from build123d import *

# Parameters (mm, degrees)
BOSS_EXTRUDE1_DEPTH            = 7.5
M3_CLEARANCE_HOLE1_D           = 3.4
M3_CLEARANCE_HOLE1_CSINK_D     = 3.45
M3_CLEARANCE_HOLE1_CSINK_ANGLE = 90
FILLET1_R                      = 30


with BuildPart() as part:
    # Sketch1 → Boss-Extrude1 (new body)
    with BuildSketch(Plane(origin=(0, 0, 0), x_dir=(0, 0, -1), z_dir=(1, 0, 0))):
        Polygon((0, 0), (0, 45), (9.5, 45), (9.5, 9.5), (40, 9.5), (40, 0), align=None)
    extrude(amount=BOSS_EXTRUDE1_DEPTH)

    # M3 Clearance Hole1 (through all)
    with Locations(Plane(origin=(7.5, 0, 0), x_dir=(0, 0, -1), z_dir=(1, 0, 0))):
        with Locations((35, 5), (10, 5), (5, 39.5), (5, 14.5)):
            CounterSinkHole(M3_CLEARANCE_HOLE1_D / 2, M3_CLEARANCE_HOLE1_CSINK_D / 2, counter_sink_angle=M3_CLEARANCE_HOLE1_CSINK_ANGLE)

    # Fillet1
    fillet1_edges = [part.edges().sort_by_distance(p)[0] for p in [
        (3.75, 9.5, -9.5),
    ]]
    fillet(fillet1_edges, radius=FILLET1_R)


solid = part.part
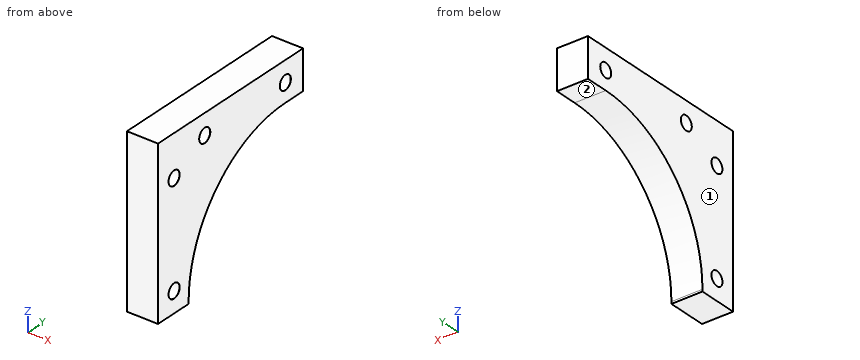
Source: CAD feature listing. Evaluate the final solid. Frame: model axes, mm. Face numbers are marked on the shaded views. A direction names the side the tool comes from. Round coordinates to 2 decimals unless told otherwise and drop trailing zeros. Order: outer loops, then holes, each group sorted by start corner. A loop starts at its lowest first (then second) coordinate and runs counter-clockwise, first axis right, second up. Notation, with made-up numbers: (51.25, -11) - (94.25, -11) arc R21 ccw to (94.25, -4) - close; hole circle Ø7 at (88.5, -39). An arc over 180 degrees is marked (long way). Use a Markdown table: item, result. Add a question column.
1. Set-up query: the marked faces 1 and 2. Return all of +Z, -Z, +X, -X, +Y, -Y with unobstructed straight access to the full face (end or side cutting, diameter ignored); none if empty.
2. Section query D-D (y = 14.5). Return the cut outline in (x, z) (3 decimals).
3. Section query C-C (z = -35). Return the cut outline in (x, y) (3 decimals), then the cut area to 3 significant figures.
4. Line query: probe 1 along Y at (x, z) = (5.75, -5); probe 2 along Z at (x, y) = (3.5, 5); probe 3 along Z at (x, y) = (5.25, 39.5). Output: solid intervals per line, ascending.
5. First-contact query: pin 1 (2 mm diameter, centred on y = 5, z = -35, fed in from -X); pin 2 (1 mm diameter, centred on x = 4.5, z = -25, fed in from +Y). Flat tips, straight axial feed; report the tip coordinate or a pass-through.
6. Section query B-B (x = 2.75). Return the cut outline in (y, z).
7. Section query A-A (y = 5). Return the cut outline in (x, z) (3 decimals), then the cut area to 3 significant figures.
Derived:
| question | item | result |
|---|---|---|
| 1 | face 1 | +Z, -Z, -X, +Y, -Y |
| 1 | face 2 | -Z, +X, -X, +Y |
| 2 | outline | (0, -22.917) - (7.5, -22.917) - (7.5, -6.725) - (7.475, -6.7) - (0, -6.7) - close; (0, -3.3) - (7.475, -3.3) - (7.5, -3.275) - (7.5, 0) - (0, 0) - close |
| 3 | outline | (0, 0) - (7.5, 0) - (7.5, 3.275) - (7.475, 3.3) - (0, 3.3) - close; (0, 6.7) - (7.475, 6.7) - (7.5, 6.725) - (7.5, 9.839) - (0, 9.839) - close |
| 3 | area | 48.3 mm2 |
| 4 | probe 1 | 0 to 12.8, 16.2 to 37.8, 41.2 to 45 |
| 4 | probe 2 | -40 to -36.7, -33.3 to -11.7, -8.3 to 0 |
| 4 | probe 3 | -9.5 to -6.7, -3.3 to 0 |
| 5 | pin 1 | through |
| 5 | pin 2 | y = 13.52 |
| 6 | outline | (0, -40) - (9.5, -40) - (9.5, -39.5) arc R30 cw to (39.5, -9.5) - (45, -9.5) - (45, 0) - (0, 0) - close; hole circle Ø3.4 at (5, -35); hole circle Ø3.4 at (5, -10); hole circle Ø3.4 at (14.5, -5); hole circle Ø3.4 at (39.5, -5) |
| 7 | outline | (0, -40) - (7.5, -40) - (7.5, -36.725) - (7.475, -36.7) - (0, -36.7) - close; (0, -33.3) - (7.475, -33.3) - (7.5, -33.275) - (7.5, -11.725) - (7.475, -11.7) - (0, -11.7) - close; (0, -8.3) - (7.475, -8.3) - (7.5, -8.275) - (7.5, 0) - (0, 0) - close |
| 7 | area | 249 mm2 |
